Could you check a few things on this model? Use its own coordinates, in mm. A direction names the side the tool comes from. Round coordinates to 2 decimals unless told otherwise and drop trailing zeros. Write each loop counter-clockwise with the first axis right and the second up, starting at its lowest first coordinate (ties: lowest second). Pieces come first, ordered by that corner, then holes. Notation, with made-up numbers: M 48.5,-37 L 83.5,-37 A16 cw 83.5,-26 Z; hole C -18.75,-37 d9. An arc over 180 degrees is marked long. One line per question, with ' | ' between items. Start each with the question number.
```python
from build123d import *

# Parameters (mm, degrees)
SKETCH_1_W          = 42.3
SKETCH_1_H          = 42.3
EXTRUDE_1_DEPTH     = 34
CHAMFER_1_SIZE      = 4.2
SKETCH_2_R          = 1.5
CUT_EXTRUDE_1_DEPTH = 4.5
SKETCH_3_R          = 11
EXTRUDE_2_DEPTH     = 2
SKETCH_4_R          = 2.5
EXTRUDE_3_DEPTH     = 20.5
CUT_EXTRUDE_2_DEPTH = 18
SKETCH_6_W          = 16
SKETCH_6_H          = 10
SKETCH_6_W_2        = 13
SKETCH_6_H_2        = 6
EXTRUDE_4_DEPTH     = 7
SKETCH_7_W          = 23
SKETCH_7_H          = 6
EXTRUDE_5_DEPTH     = 8


with BuildPart() as part:
    # 草图1 → 凸台-拉伸1 (new body)
    with BuildSketch(Plane(origin=(0, 0, 0), x_dir=(1, 0, 0), z_dir=(0, 1, 0))):
        with Locations((21.15, 21.15)):
            Rectangle(SKETCH_1_W, SKETCH_1_H)
    extrude(amount=EXTRUDE_1_DEPTH)

    # 倒角1
    chamfer_1_edges = [part.edges().sort_by_distance(p)[0] for p in [
        (0, 17, -42.3),
        (42.3, 17, -42.3),
        (42.3, 17, 0),
        (0, 17, 0),
    ]]
    chamfer(chamfer_1_edges, length=CHAMFER_1_SIZE)

    # 草图2 → 切除-拉伸1 (cut)
    with BuildSketch(Plane(origin=(0, 34, 0), x_dir=(1, 0, 0), z_dir=(0, 1, 0))):
        with Locations((5.65, 36.65)):
            Circle(SKETCH_2_R)
        with Locations((36.65, 36.65)):
            Circle(SKETCH_2_R)
        with Locations((5.65, 5.65)):
            Circle(SKETCH_2_R)
        with Locations((36.65, 5.65)):
            Circle(SKETCH_2_R)
    extrude(amount=-CUT_EXTRUDE_1_DEPTH, mode=Mode.SUBTRACT)

    # 草图3 → 凸台-拉伸2 (add)
    with BuildSketch(Plane(origin=(0, 34, 0), x_dir=(1, 0, 0), z_dir=(0, 1, 0))):
        with Locations((21.15, 21.15)):
            Circle(SKETCH_3_R)
    extrude(amount=EXTRUDE_2_DEPTH)

    # 草图4 → 凸台-拉伸3 (add)
    with BuildSketch(Plane(origin=(0, 36, 0), x_dir=(1, 0, 0), z_dir=(0, 1, 0))):
        with Locations((21.15, 21.15)):
            Circle(SKETCH_4_R)
    extrude(amount=EXTRUDE_3_DEPTH)

    # 草图5 → 切除-拉伸2 (cut)
    with BuildSketch(Plane(origin=(0, 56.5, 0), x_dir=(1, 0, 0), z_dir=(0, 1, 0))):
        with BuildLine():
            Line((19.65, 23.15), (22.65, 23.15))
            ThreePointArc((22.65, 23.15), (21.15, 23.65), (19.65, 23.15))
        make_face()
    extrude(amount=-CUT_EXTRUDE_2_DEPTH, mode=Mode.SUBTRACT)

    # 草图6 → 凸台-拉伸4 (add)
    with BuildSketch(Plane.XY):
        with Locations((21.15, 15)):
            Rectangle(SKETCH_6_W, SKETCH_6_H)
        with Locations((21.15, 3)):
            Rectangle(SKETCH_6_W_2, SKETCH_6_H_2)
    extrude(amount=EXTRUDE_4_DEPTH)

    # 草图7 → 凸台-拉伸5 (add)
    with BuildSketch(Plane(origin=(42.3, 0, 0), x_dir=(0, 0, -1), z_dir=(1, 0, 0))):
        with Locations((21.15, 3)):
            Rectangle(SKETCH_7_W, SKETCH_7_H)
    extrude(amount=EXTRUDE_5_DEPTH)


solid = part.part
```
1. Suppose I cut it at A-A (y = 14.5). Write out the boundary of the cut face in (x, z).
2. I need wall thicknesses on line 1 along X through (y, z) = (32.6, -36.65); line 2 along Z through (x, y) = (36.65, 31.3); line 3 along Z through (x, y) = (5, 31). Which ranges of each line are inside material? Lowest first, please. Write a range as from..to.
3. If we mould it in two halves opening along X, with no side actions, what happens to faces 1 (the face through (21, 3, 7)), 2 (the face through (2.1, 16.8, -40.2)), 3 (the face through (37.3, 31.8, -35.3))? For each: released by +X, released by -X, zero draft, split by the parting line, or undercut.
4. Suppose I cut it at D-D (y = 31.5). Write out the boundary of the cut face in (x, z).
5. I'm going to push flat-ended pins straight in: P1, Ø3.5, axis at x = 18.5, z = 4, coming from the +Y side; P2, Ø2.5, axis at x = 5.65, z = -36.65, coming from the +Y side; P3, Ø6.5, axis at x = 47.5, y = 4.5, coming from the +Z side. Where does each tip first touch, or does it pass through?
6. Which directions (+Z, -Z, +X, -X, +Y, -Y) give clear straight access to the entire face, cutting with the end or side of a thin tool? Please do faces 4 (the face through (14.65, 3, 3)), 5 (the face through (37, 29.5, -37)), 6 (the face through (13.15, 15, 3)), 7 (the face through (46, 3, -9.65)).
7. Suppose I cut it at C-C (z = -5.65). Write out the boundary of the cut face in (x, y), and give its area (3 significant figures).
8. Suppose I cut it at B-B (x = 21.15). Write out the boundary of the cut face in (y, z).
Computed:
1) outline: M 0,-38.1 L 4.2,-42.3 L 38.1,-42.3 L 42.3,-38.1 L 42.3,-4.2 L 38.1,0 L 29.15,0 L 29.15,7 L 13.15,7 L 13.15,0 L 4.2,0 L 0,-4.2 Z
2) line 1: x = 0..4.15, 7.15..35.15, 38.15..42.3 | line 2: z = -42.3..-38.15, -35.15..-7.15, -4.15..0 | line 3: z = -42.3..-38, -35.3..-7, -4.3..0
3) face 1: zero draft | face 2: released by -X | face 3: undercut
4) outline: M 0,-38.1 L 4.2,-42.3 L 38.1,-42.3 L 42.3,-38.1 L 42.3,-4.2 L 38.1,0 L 4.2,0 L 0,-4.2 Z; hole C 5.65,-36.65 d3; hole C 5.65,-5.65 d3; hole C 36.65,-36.65 d3; hole C 36.65,-5.65 d3
5) P1: stops at y = 20 | P2: stops at y = 29.5 | P3: stops at z = -9.65
6) face 4: +Z, -X, -Y | face 5: +Y | face 6: +Z, -X, +Y, -Y | face 7: +Z, +X, +Y, -Y
7) outline: M 0,0 L 42.3,0 L 42.3,34 L 38.15,34 L 38.15,29.5 L 35.15,29.5 L 35.15,34 L 7.15,34 L 7.15,29.5 L 4.15,29.5 L 4.15,34 L 0,34 Z | area: 1,410 mm²
8) outline: M 0,-42.3 L 34,-42.3 L 34,-32.15 L 36,-32.15 L 36,-23.65 L 38.5,-23.65 L 38.5,-23.15 L 56.5,-23.15 L 56.5,-18.65 L 36,-18.65 L 36,-10.15 L 34,-10.15 L 34,0 L 20,0 L 20,7 L 10,7 L 10,0 L 6,0 L 6,7 L 0,7 Z
